Can you work these out from the drawing? Everything is in mm from the part's minimum corner. A direction names the side the tool comes from. Coordinates: 2 decimals unless noted, no trailing zeros. Loops run counter-clockwise (first coordinate to the right, second up) from the corner with the lowest first, then second, coordinate; pieces in that order, holes last. Notation, with made-up numbers: (45.5, 55) -> (93.5, 55) arc R12 ccw to (93.5, 71) -> close; hole circle Ø3 at (-10, 79.5). An arc over 180 degrees is marked (long way). Use one line per item in the form item = value. Start each with the question number.
(1) Imagine slicing it at A-A (z = 24.25). List the corners of the cut face in (x, y) for me, plus the area to 3 significant figures.
(2) Imagine slicing it at B-B (x = 30). List the corners of the cut face in (y, z) for me, plus the area to 3 significant figures.
(3) I'm going to push flat-ended pins straight in: pin 1 (5 mm diameter, centred on y = 18, z = 3.5, fed in from -X); pin 2 (10 mm diameter, centred on y = 41.5, z = 4.5, fed in from -X); pin 3 (2 mm diameter, centred on x = 149, z = 5, fed in from -Y). Where does each tip first touch, or does it pass through?
(4) Imagine slicing it at C-C (y = 30). List the corners of the cut face in (x, z) for me.
(5) Thinking about a two-plate mould opening in X: for the marked faces 1 and 2, which applies, released by +X, released by -X, zero draft, split by the parting line, or undercut?
(6) On a 3-axis mill with a long thin cutter (end or side, diameter ignored), from which of +Z, -Z, +X, -X, +Y, -Y can I reach the whole of each face in a straight line? I mean the marked faces 3, 4 and 5. Say none if no direction works.
(7) Imagine slicing it at D-D (x = 140). List the corners of the cut face in (y, z) for me.
(8) I need wall thicknesses on line 1 (Y direction, x = 30, z = 23); line 2 (Y direction, x = 114, z = 11.75); line 3 (X direction, y = 5.5, z = 21). Which ranges of each line are inside material? Lowest first, please. Write a range as [from, to].
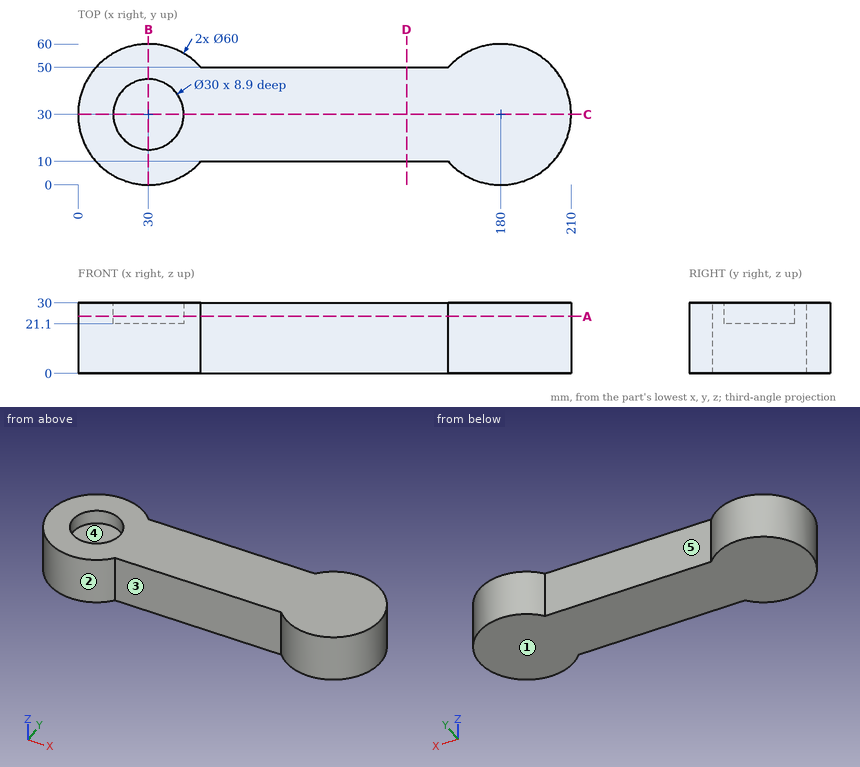
Worked out:
q1.outline = (52.36, 10) -> (157.64, 10) arc R30 ccw (long way) to (157.64, 50) -> (52.36, 50) arc R30 ccw (long way) to start; hole circle Ø30 at (30, 30)
q1.area = 8,740 mm2
q2.outline = (0, 0) -> (60, 0) -> (60, 30) -> (45, 30) -> (45, 21.1) -> (15, 21.1) -> (15, 30) -> (0, 30) -> close
q2.area = 1,530 mm2
q3.pin_1 = 1.54
q3.pin_2 = 0.71
q3.pin_3 = 10
q4.outline = (0, 0) -> (210, 0) -> (210, 30) -> (45, 30) -> (45, 21.1) -> (15, 21.1) -> (15, 30) -> (0, 30) -> close
q5.face_1 = zero draft
q5.face_2 = undercut
q6.face_3 = +Z, -Z, -Y
q6.face_4 = +Z
q6.face_5 = +Z, -Z, +Y
q7.outline = (10, 0) -> (50, 0) -> (50, 30) -> (10, 30) -> close
q8.line_1 = [0, 15], [45, 60]
q8.line_2 = [10, 50]
q8.line_3 = [12.69, 47.31], [162.69, 197.31]
